```python
from build123d import *

# Parameters (mm, degrees)
CYLINDER003_R     = 2
CYLINDER003_DEPTH = 10
CYLINDER004_R     = 2
CYLINDER004_DEPTH = 30
CYLINDER001_R     = 10.2
CYLINDER001_DEPTH = 10
BOX_W             = 10
BOX_H             = 25
BOX_DEPTH         = 10
CYLINDER_R        = 15
CYLINDER_DEPTH    = 10


with BuildPart() as cylinder003:
    # Cylinder003 → Cylinder003 (new body)
    with BuildSketch(Plane(origin=(15, 20, 0), x_dir=(0, 0, 1), z_dir=(-1, 0, 0))):
        Circle(CYLINDER003_R)
    extrude(amount=CYLINDER003_DEPTH)


with BuildPart() as cylinder004:
    # Cylinder004 → Cylinder004 (new body)
    with BuildSketch(Plane.ZY.offset(-15)):
        Circle(CYLINDER004_R)
    extrude(amount=CYLINDER004_DEPTH)


with BuildPart() as negative_fusion:
    # Cylinder001 → Cylinder001 (new body)
    with BuildSketch(Plane.XY.offset(-5)):
        Circle(CYLINDER001_R)
    extrude(amount=CYLINDER001_DEPTH)

    # Fusion: union Cylinder003, Cylinder004
    add(cylinder003.part)
    add(cylinder004.part)


with BuildPart() as cube:
    # Box → Box (new body)
    with BuildSketch(Plane(origin=(5, 0, -5), x_dir=(1, 0, 0), z_dir=(0, 0, 1))):
        with Locations((5, 12.5)):
            Rectangle(BOX_W, BOX_H)
    extrude(amount=BOX_DEPTH)


with BuildPart() as cut:
    # Cylinder → Cylinder (new body)
    with BuildSketch(Plane.XY.offset(-5)):
        Circle(CYLINDER_R)
    extrude(amount=CYLINDER_DEPTH)

    # Fusion001: union Cube
    add(cube.part)

    # Cut: cut Negative Fusion
    add(negative_fusion.part, mode=Mode.SUBTRACT)


solid = cut.part
```
Work out the finished part from the listing and answer in its coordinate system (mm). A direction names the side the tool comes from. Coordinates: 2 decimals unless noted, no trailing zeros. Loops run counter-clockwise (first coordinate to the right, second up) from the corner with the lowest first, then second, coordinate; pieces in that order, holes last. Notation, with made-up numbers: (66, 23.25) -> (111, 23.25) arc R26 cw to (111, 38.25) -> close; hole circle Ø9 at (4.5, 79.5). An arc over 180 degrees is marked (long way). Answer as CSV lines item,"result".
Q1. The part is cut by section D-D on z = -3.5. Write down the section's boundary in (x, y), and give its area (3 significant figures).
Findings:
outline,"(5, 14.14) arc R15 ccw (long way) to (15, 0) -> (15, 25) -> (5, 25) -> close; hole circle Ø20.4 at (0, 0)"
area,"527 mm²"
Q2. The part is cut by section C-C on x = 0. Write down the section's boundary in (y, z), and give its area (3 significant figures).
Findings:
outline,"(-15, -5) -> (-10.2, -5) -> (-10.2, 5) -> (-15, 5) -> close; (10.2, -5) -> (15, -5) -> (15, 5) -> (10.2, 5) -> close"
area,"96.0 mm²"
Q3. The part is cut by section B-B on z = -0.75. Write down the section's boundary in (x, y).
Findings:
outline,"(-14.88, -1.85) arc R15 ccw to (14.88, -1.85) -> (10.03, -1.85) arc R10.2 cw to (-10.03, -1.85) -> close; (-14.88, 1.85) -> (-10.03, 1.85) arc R10.2 cw to (10.03, 1.85) -> (15, 1.85) -> (15, 18.15) -> (5, 18.15) -> (5, 14.14) arc R15 ccw to start; (5, 21.85) -> (15, 21.85) -> (15, 25) -> (5, 25) -> close"
Q4. For a pull along X with two mould halves and no side action, classify faces 1 (the face through (10, 25, 0)), 2 (the face through (15, 12, 0)), 3 (the face through (9.73, 3.06, -0.07)) as +X half, -X half, draft (parallel to the pull), parting line (faces both ways), or undercut.
Findings:
face 1,"draft"
face 2,"+X half"
face 3,"undercut"
Q5. Each of these flat-tipped pins is pushed along its axis until it touches: pin 1 (1.5 mm diameter, centred on y = 16.5, z = -1.5, fed in from -X); pin 2 (1.5 mm diameter, centred on y = 9, z = 1, fed in from -X); pin 3 (1 mm diameter, centred on x = 2, z = 3, fed in from +Y); pin 4 (2.5 mm diameter, centred on y = 20, z = 0, fed in from -X). Where does it stop, or does it pass through?
Findings:
pin 1,"stops at x = 5"
pin 2,"stops at x = -12.53"
pin 3,"stops at y = 14.92"
pin 4,"passes through"
Q6. A tool of negligible diameter and unlimited length cuts with its end or side. For faces 4 (the face through (5, 18, 1)), 5 (the face through (10, 22, 0)), from which of +Z, -Z, +X, -X, +Y, -Y can it reach the whole face along a straight path? Write none if from no direction.
Findings:
face 4,"+Z, -Z, +Y"
face 5,"+X, -X"
Q7. The part is cut by section A-A on y = 20. Write down the section's boundary in (x, z).
Findings:
outline,"(5, -5) -> (15, -5) -> (15, -2) -> (5, -2) -> close; (5, 2) -> (15, 2) -> (15, 5) -> (5, 5) -> close"
Q8. Find the intervals of material crossed by probe 1 along Z at (x, y) = (12.4, 0); probe 2 along Y at (x, z) = (0, -2.25); probe 3 along X at (y, z) = (16, 2.5), in increasing order.
Findings:
probe 1,"z = -5 to -2, 2 to 5"
probe 2,"y = -15 to -10.2, 10.2 to 15"
probe 3,"x = 5 to 15"
